Autodesk Inventor part; units mm, degrees
ref_plane "YZ Plane" through (0, 0, 0) normal (1, 0, 0) x (0, 1, 0)
ref_plane "XZ Plane" through (0, 0, 0) normal (0, 1, 0) x (-1, 0, 0)
ref_plane "XY Plane" through (0, 0, 0) normal (0, 0, 1) x (1, 0, 0)
sketch "스케치1" plane through (0, 0, 0) normal (1, 0, 0) x (0, 1, 0)
  circle A0 centre (0, 0) radius 8.45
  dimension "d0" = 16.9
extrude "돌출1" add sketch "스케치1" along normal blind 15
sketch "스케치2" plane through (15, 0, 0) normal (1, 0, 0) x (0, 0, -1)
  circle A0 centre (0, 0) radius 2.5
  line L0 (-2.4495, 0.5) -> (2.4495, 0.5)
  line L1 (-2.4495, -0.5) -> (2.4495, -0.5)
  point P0 (0, 0.5)
  dimension "d3" = 5
  dimension "d4" = 1
  dimension "d5" = 0.5
extrude "돌출2" add sketch "스케치2" along normal blind 10 contours L0 A0 | A0 L1
sketch "스케치3" plane through (0, 0, 0) normal (-1, 0, 0) x (0, 0, 1)
  line L0 (-7.5, -3.8926) -> (7.5, -3.8926)
  line L1 (7.5, -3.8926) -> (7.5, -9.8926)
  line L2 (7.5, -9.8926) -> (-7.5, -9.8926)
  line L3 (-7.5, -9.8926) -> (-7.5, -3.8926)
  circle A0 centre (0, 0) radius 8.45
  line L4 (-5.0426, -9.8926) -> (-3.5426, -9.8926)
  line L5 (-3.5426, -9.8926) -> (-3.5426, -13.8926)
  line L6 (-3.5426, -13.8926) -> (-5.0426, -13.8926)
  line L7 (-5.0426, -13.8926) -> (-5.0426, -9.8926)
  line L8 (-0.7464, -9.8926) -> (0.7536, -9.8926)
  line L9 (0.7536, -9.8926) -> (0.7536, -13.8926)
  line L10 (0.7536, -13.8926) -> (-0.7464, -13.8926)
  line L11 (-0.7464, -13.8926) -> (-0.7464, -9.8926)
  line L12 (3.4319, -9.8926) -> (4.9319, -9.8926)
  line L13 (4.9319, -9.8926) -> (4.9319, -13.8926)
  line L14 (4.9319, -13.8926) -> (3.4319, -13.8926)
  line L15 (3.4319, -13.8926) -> (3.4319, -9.8926)
  point P0 (0.7536, -9.8926)
  dimension "d8" = 6
  dimension "d9" = 15
  dimension "d10" = 4
  dimension "d11" = 4
  dimension "d12" = 1.5
  dimension "d13" = 1.5
  dimension "d14" = 1.5
extrude "돌출3" add sketch "스케치3" against normal blind 15 contours A0 L1 L2 L3 | L2 L5 L6 L7 | L13 L14 L15 L2 | L2 L9 L10 L11
equation "\"d11\" = d10"
equation "\"d13\" = d12"
equation "\"d14\" = d12"
properties part number "가변저항"
CAD build for the part. Positions are in the model's coordinates, mm. A direction names the side the tool comes from. Give positions to 0.01 mm unless a question says otherwise; leave off trailing zeros. Order: outer loops, then holes, each group sorted by start corner. A loop starts at its lowest first (then second) coordinate and runs counter-clockwise, first axis right, second up.
(1) Saw through at D-D, the plane x = 17.5. Give the cut face in (y, z), then the cut area to 3 significant figures.
(2) Drill centre lines: L1, parallel to Z at x = 7.75, y = -10; L2, parallel to Z at x = 8, y = -5; L3, parallel to X at y = -2.5, z = -6. Where is each one in solid material? Low to high.
(3) Mould opens along Y. For faces 4 (the flat face through (20, 0.5, 0)), 5 (the flat face through (25, 1, 0)), 6 (the flat face through (7, -9.893, -2)) say: released by +Y, released by -Y, zero draft, split by the parting line, or undercut.
(4) Saw through at B-B, the plane z = 0. Give the cut face in (x, y), then the cut area to 3 significant figures.
(5) Saw through at A-A, the plane y = -10.25. Give the cut face in (x, z), then the cut area to 3 significant figures.
(6) Tool access for faces 1 (the cylindrical face through (19.9, 2.5, 0)), 2 (the flat face through (7, -7, 7.5)), 3 (the cylindrical face through (19.9, -2.5, 0)): list every direction of +Z, -Z, +X, -X, +Y, -Y with a clear straight run to the whole face (end or side of a thin tool).
(7) Flat gauge pins, fed straight in: pin 1 (4.5 mm diameter, centred on x = 9, y = -11, fed in from -Z); pin 2 (6 mm diameter, centred on x = 14.5, z = 3.5, fed in from +Y); pin 3 (4 mm diameter, centred on x = 19, y = 1, fed in from +Z). Where does each tip first touch, or does it go through?
(8) Saw through at C-C, the plane x = 14.5. Give the cut face in (y, z), then the cut area to 3 significant figures.
Results found:
1. outline: (-0.5, -2.45) - (-0.5, 2.45) arc R2.5 ccw to start; (0.5, -2.45) arc R2.5 ccw to (0.5, 2.45) - close
1. area: 14.7 mm2
2. L1: z = -5.04 to -3.54, -0.75 to 0.75, 3.43 to 4.93
2. L2: z = -7.5 to 7.5
2. L3: x = 0 to 15
3. face 4: undercut
3. face 5: zero draft
3. face 6: released by -Y
4. outline: (0, -13.89) - (15, -13.89) - (15, -2.5) - (25, -2.5) - (25, -0.5) - (15, -0.5) - (15, 0.5) - (25, 0.5) - (25, 2.5) - (15, 2.5) - (15, 8.45) - (0, 8.45) - close
4. area: 375 mm2
5. outline: (0, -5.04) - (15, -5.04) - (15, -3.54) - (0, -3.54) - close; (0, -0.75) - (15, -0.75) - (15, 0.75) - (0, 0.75) - close; (0, 3.43) - (15, 3.43) - (15, 4.93) - (0, 4.93) - close
5. area: 67.5 mm2
6. face 1: +X, +Y
6. face 2: +Z, +X, -X, -Y
6. face 3: +X, -Y
7. pin 1: stops at z = -7.5
7. pin 2: stops at y = 8.44
7. pin 3: stops at z = 2.45
8. outline: (-13.89, -5.04) - (-9.89, -5.04) - (-9.89, -7.5) - (-3.89, -7.5) arc R8.45 ccw (long way) to (-3.89, 7.5) - (-9.89, 7.5) - (-9.89, 4.93) - (-13.89, 4.93) - (-13.89, 3.43) - (-9.89, 3.43) - (-9.89, 0.75) - (-13.89, 0.75) - (-13.89, -0.75) - (-9.89, -0.75) - (-9.89, -3.54) - (-13.89, -3.54) - close
8. area: 284 mm2
